from build123d import *

# Parameters (mm, degrees)
SKETCH1_W               = 101.6
SKETCH1_H               = 76.2
BOSS_EXTRUDE1_DEPTH     = 19.05
SKETCH2_W               = 38.1
SKETCH2_H               = 50.8
CUT_EXTRUDE1_DEPTH      = 6.35
SKETCH3_W               = 25.4
SKETCH3_H               = 2.54
CUT_EXTRUDE2_DEPTH      = 94.541341128
CHAMFER1_SIZE           = 2.54
SKETCH4_R               = 0.762
CUT_EXTRUDE3_DEPTH      = 6.35
LPATTERN1_COUNT         = 8
LPATTERN1_PITCH         = 6.35
MIRROR1_COPY_1_SKETCH_R = 0.762
MIRROR1_COPY_1_DEPTH    = 6.35
MIRROR1_COPY_2_SKETCH_R = 0.762
MIRROR1_COPY_2_DEPTH    = 6.35
MIRROR1_COPY_3_SKETCH_R = 0.762
MIRROR1_COPY_3_DEPTH    = 6.35
MIRROR1_COPY_4_SKETCH_R = 0.762
MIRROR1_COPY_4_DEPTH    = 6.35
MIRROR1_COPY_5_SKETCH_R = 0.762
MIRROR1_COPY_5_DEPTH    = 6.35
MIRROR1_COPY_6_SKETCH_R = 0.762
MIRROR1_COPY_6_DEPTH    = 6.35
MIRROR1_COPY_7_SKETCH_R = 0.762
MIRROR1_COPY_7_DEPTH    = 6.35
SKETCH6_W               = 0.762
SKETCH6_H               = 1.016
CUT_EXTRUDE8_DEPTH      = 111.168382488
LPATTERN2_COUNT         = 8
LPATTERN2_PITCH         = 3.048


with BuildPart() as part:
    # Sketch1 → Boss-Extrude1 (new body)
    with BuildSketch(Plane(origin=(0, 0, 0), x_dir=(1, 0, 0), z_dir=(0, 1, 0))):
        Rectangle(SKETCH1_W, SKETCH1_H)
    extrude(amount=BOSS_EXTRUDE1_DEPTH)

    # Sketch2 → Cut-Extrude1 (cut)
    with BuildSketch(Plane(origin=(0, 19.05, 0), x_dir=(1, 0, 0), z_dir=(0, 1, 0))):
        Rectangle(SKETCH2_W, SKETCH2_H)
    extrude(amount=-CUT_EXTRUDE1_DEPTH, mode=Mode.SUBTRACT)

    # Sketch3 → Cut-Extrude2 (cut, through all)
    with BuildSketch(Plane.XY.offset(38.1)):
        with Locations((-38.1, 17.78)):
            Rectangle(SKETCH3_W, SKETCH3_H)
        with Locations((38.1, 17.78)):
            Rectangle(SKETCH3_W, SKETCH3_H)
    extrude(amount=-CUT_EXTRUDE2_DEPTH, mode=Mode.SUBTRACT)

    # Chamfer1
    chamfer1_edges = [part.edges().sort_by_distance(p)[0] for p in [
        (25.4, 19.05, 0),
        (-25.4, 19.05, 0),
        (0, 19.05, -38.1),
        (0, 19.05, 38.1),
    ]]
    chamfer(chamfer1_edges, length=CHAMFER1_SIZE - 0.0001)  # a hair under: the kernel refuses the full size

    # Sketch4 → Cut-Extrude3 (cut)
    with BuildSketch(Plane(origin=(0, 16.51, 0), x_dir=(1, 0, 0), z_dir=(0, 1, 0))):
        with Locations(Location((-43.18, 22.225, 0), (0, 0, 270))):
            Circle(SKETCH4_R)
    cut_extrude3 = extrude(amount=-CUT_EXTRUDE3_DEPTH, mode=Mode.SUBTRACT)

    # LPattern1: Cut-Extrude3 ×8
    with Locations(*[(0, 0, i * LPATTERN1_PITCH) for i in range(1, LPATTERN1_COUNT)]):
        add(cut_extrude3, mode=Mode.SUBTRACT)

    # Mirror1: Cut-Extrude3 across plane
    add(cut_extrude3.mirror(Plane(origin=(0, 0, 0), x_dir=(0, 0, 1), z_dir=(1, 0, 0))), mode=Mode.SUBTRACT)

    # Mirror1 copy 1 sketch → Mirror1 copy 1 (cut)
    with BuildSketch(Plane(origin=(0, 16.51, 6.35), x_dir=(-1, 0, 0), z_dir=(0, 1, 0))):
        with Locations((-43.18, -22.225)):
            Circle(MIRROR1_COPY_1_SKETCH_R)
    extrude(amount=-MIRROR1_COPY_1_DEPTH, mode=Mode.SUBTRACT)

    # Mirror1 copy 2 sketch → Mirror1 copy 2 (cut)
    with BuildSketch(Plane(origin=(0, 16.51, 12.7), x_dir=(-1, 0, 0), z_dir=(0, 1, 0))):
        with Locations((-43.18, -22.225)):
            Circle(MIRROR1_COPY_2_SKETCH_R)
    extrude(amount=-MIRROR1_COPY_2_DEPTH, mode=Mode.SUBTRACT)

    # Mirror1 copy 3 sketch → Mirror1 copy 3 (cut)
    with BuildSketch(Plane(origin=(0, 16.51, 19.05), x_dir=(-1, 0, 0), z_dir=(0, 1, 0))):
        with Locations((-43.18, -22.225)):
            Circle(MIRROR1_COPY_3_SKETCH_R)
    extrude(amount=-MIRROR1_COPY_3_DEPTH, mode=Mode.SUBTRACT)

    # Mirror1 copy 4 sketch → Mirror1 copy 4 (cut)
    with BuildSketch(Plane(origin=(0, 16.51, 25.4), x_dir=(-1, 0, 0), z_dir=(0, 1, 0))):
        with Locations((-43.18, -22.225)):
            Circle(MIRROR1_COPY_4_SKETCH_R)
    extrude(amount=-MIRROR1_COPY_4_DEPTH, mode=Mode.SUBTRACT)

    # Mirror1 copy 5 sketch → Mirror1 copy 5 (cut)
    with BuildSketch(Plane(origin=(0, 16.51, 31.75), x_dir=(-1, 0, 0), z_dir=(0, 1, 0))):
        with Locations((-43.18, -22.225)):
            Circle(MIRROR1_COPY_5_SKETCH_R)
    extrude(amount=-MIRROR1_COPY_5_DEPTH, mode=Mode.SUBTRACT)

    # Mirror1 copy 6 sketch → Mirror1 copy 6 (cut)
    with BuildSketch(Plane(origin=(0, 16.51, 38.1), x_dir=(-1, 0, 0), z_dir=(0, 1, 0))):
        with Locations((-43.18, -22.225)):
            Circle(MIRROR1_COPY_6_SKETCH_R)
    extrude(amount=-MIRROR1_COPY_6_DEPTH, mode=Mode.SUBTRACT)

    # Mirror1 copy 7 sketch → Mirror1 copy 7 (cut)
    with BuildSketch(Plane(origin=(0, 16.51, 44.45), x_dir=(-1, 0, 0), z_dir=(0, 1, 0))):
        with Locations((-43.18, -22.225)):
            Circle(MIRROR1_COPY_7_SKETCH_R)
    extrude(amount=-MIRROR1_COPY_7_DEPTH, mode=Mode.SUBTRACT)

    # Sketch6 → Cut-Extrude8 (cut, through all)
    with BuildSketch(Plane.ZY.offset(50.8)):
        with Locations((-10.668, 18.542)):
            Rectangle(SKETCH6_W, SKETCH6_H)
    cut_extrude8 = extrude(amount=-CUT_EXTRUDE8_DEPTH, mode=Mode.SUBTRACT)

    # LPattern2: Cut-Extrude8 ×8
    with Locations(*[(0, 0, i * LPATTERN2_PITCH) for i in range(1, LPATTERN2_COUNT)]):
        add(cut_extrude8, mode=Mode.SUBTRACT)


solid = part.part
Could you check a few things on this model? Use its own coordinates, in mm. A direction names the side the tool comes from. Give positions to 0.01 mm unless a question says otherwise; leave off trailing zeros. Loops run counter-clockwise (first coordinate to the right, second up) from the corner with the lowest first, then second, coordinate; pieces in that order, holes last. Notation, with made-up numbers: (25, 20) -> (44, 20) arc R26 ccw to (44, 34) -> close; hole circle Ø6 at (-17.75, 0.5). An arc over 180 degrees is marked (long way). Return JSON: item names as keys, results as strings.
Item 1: I need wall thicknesses on L1, parallel to X at y = 11.75, z = 10; L2, parallel to X at y = 14.25, z = 4; L3, parallel to Y at x = 46.5, z = 23. Which ranges of each line are inside material? Lowest first, please. Write a range as from..to.
Geometry results:
{"L1": "x = -50.8..-43.78, -42.58..42.58, 43.78..50.8", "L2": "x = -50.8..-19.05, 19.05..50.8", "L3": "y = 0..16.51"}
Item 2: I'm going to push flat-ended pins straight in: pin 1 (4 mm diameter, centred on x = -40, z = -10.5, fed in from -Y); pin 2 (2 mm diameter, centred on x = 43.18, z = 15.875, fed in from +Y); pin 3 (0.8 mm diameter, centred on x = 22, y = 18.5, fed in from -Z); pin 4 (0.5 mm diameter, centred on x = -21, y = 18.5, fed in from -Z). Where does each tip first touch, or does it pass through?
Geometry results:
{"pin 1": "stops at y = 0", "pin 2": "stops at y = 16.51", "pin 3": "stops at z = -36.51", "pin 4": "stops at z = -36.36"}
Item 3: If we section it at B-B on x = -13: List the corners of the cut face in (y, z) for me, plus the area to 3 significant figures.
Geometry results:
{"outline": "(0, -38.1) -> (16.51, -38.1) -> (19.05, -35.56) -> (19.05, -25.4) -> (12.7, -25.4) -> (12.7, 25.4) -> (19.05, 25.4) -> (19.05, 35.56) -> (16.51, 38.1) -> (0, 38.1) -> close", "area": "1,120 mm²"}
Item 4: We'd pull the mould along Z, two halves only. Please class faces 4 (the flat face through (-1, 8, 38.1)), 5 (the flat face through (-21, 19.05, -6)), 6 (the flat face through (0, 16, 25.4)): +Z half, -Z half, draft (parallel to the pull), parting line (faces both ways), or undercut.
Geometry results:
{"face 4": "+Z half", "face 5": "draft", "face 6": "undercut"}
Item 5: Which directions (+Z, -Z, +X, -X, +Y, -Y) give clear straight access to the entire face, cutting with the end or side of a thin tool? Please do faces 1 (the flat face through (38, 16.51, 1)), 2 (the flat face through (19.05, 16, 0)), 3 (the flat face through (-38, 16.51, 1)).
Geometry results:
{"face 1": "+Z, -Z, +X, +Y", "face 2": "+Y", "face 3": "+Z, -Z, -X, +Y"}
